```python
from build123d import *

# Parameters (mm, degrees)
F0_W           = 850
F0_H           = 1920
F0_W_2         = 810
F0_H_2         = 1880
F1_DEPTH       = 20
F2_W           = 850
F2_H           = 50
F3_DEPTH       = 10
F6_DEPTH       = 20
F8_DEPTH       = 10
F8_DEPTH_BACK  = 10
F10_DEPTH      = 20
F11_R          = 4.25
F12_DEPTH      = 960.001
F12_DEPTH_BACK = 960.001


with BuildPart() as f1:
    # F0 (on Top) → F1 (new body)
    with BuildSketch(Plane.XY):
        Rectangle(F0_W, F0_H)
        Rectangle(F0_W_2, F0_H_2, mode=Mode.SUBTRACT)
    extrude(amount=F1_DEPTH)

    # F2 (on face) → F3 (join)
    with BuildSketch(Plane.XY.offset(20)):
        with Locations((0, 785)):
            Rectangle(F2_W, F2_H)
        with Locations((0, 585)):
            Rectangle(F2_W, F2_H)
        with Locations((0, 385)):
            Rectangle(F2_W, F2_H)
        with Locations((0, 185)):
            Rectangle(F2_W, F2_H)
        with Locations((0, -15)):
            Rectangle(F2_W, F2_H)
        with Locations((0, -215)):
            Rectangle(F2_W, F2_H)
        with Locations((0, -415)):
            Rectangle(F2_W, F2_H)
        with Locations((0, -615)):
            Rectangle(F2_W, F2_H)
        with Locations((0, -815)):
            Rectangle(F2_W, F2_H)
    extrude(amount=F3_DEPTH)

    # F5 (on face) → F6 (join)
    with BuildSketch(Plane.XZ.offset(960)):
        Polygon((445, 180), (425, 180), (425, 0), (145, 0), (145, -20), (445, -20), align=None)
    extrude(amount=-F6_DEPTH)

    # F7 (on Front) → F8 (join, two sides)
    with BuildSketch(Plane.XZ) as f8_sk:
        Polygon((425, 0), (-425, 0), (-425, -20), (445, -20), (445, 180), (425, 180), align=None)
    extrude(amount=F8_DEPTH)
    extrude(f8_sk.sketch, amount=-F8_DEPTH_BACK)

    # F9 (on face) → F10 (join)
    with BuildSketch(Plane(origin=(0, 960, 0), x_dir=(-1, 0, 0), z_dir=(0, 1, 0))):
        Polygon((425, 0), (-425, 0), (-425, 180), (-445, 180), (-445, -20), (425, -20), align=None)
    extrude(amount=-F10_DEPTH)

    # F11 (on Front) → F12 (cut, two sides)
    with BuildSketch(Plane.XZ) as f12_sk:
        with Locations((435, 170)):
            Circle(F11_R)
    extrude(amount=-F12_DEPTH, mode=Mode.SUBTRACT)
    extrude(f12_sk.sketch, amount=F12_DEPTH_BACK, mode=Mode.SUBTRACT)


solid = f1.part
```
For this review, take the finished solid that the model builds, in its own axes (mm). A direction names the side the tool comes from. Round coordinates to 2 decimals unless told otherwise and drop trailing zeros. Write each loop counter-clockwise with the first axis right and the second up, starting at its lowest first coordinate (ties: lowest second). Pieces come first, ordered by that corner, then holes. Notation, with made-up numbers: (-1, 70.25) -> (4, 70.25) arc R14 ccw to (4, 89.25) -> close; hole circle Ø1 at (53, 11). An arc over 180 degrees is marked (long way). One line per question, with ' | ' between items. Start each with the question number.
(1) For line 1 along Z through (x, y) = (435, 4.75); line 2 along Y through (x, z) = (371.5, -8); line 3 along Y through (x, z) = (-254, -8.5), list the stretches that pass through material, from the lowest coordinate up. Write a range as from..to.
(2) Tool access review of faces 1 (the face through (-2, 941, 20)), 2 (the face through (-416, -694, 0)), 3 (the face through (-6, 185, 20)), 4 (the face through (-6, -15, 20)): name each direction out of +Z, -Z, +X, -X, +Y, -Y from which nothing blocks a thin tool from reaching the whole face with its end or side.
(3) Insertion check: P1, Ø16, axis at x = -418, y = -527, coming from the +Z side; P2, Ø3, axis at x = -35.5, z = 26.5, coming from the -Y side; P3, Ø6, axis at y = -237.5, z = 2, coming from the +X side. Each pin has a flat end and moves straight along its axis. Give the tip position at first contact, or say it passes through.
(4) Mouldability with a two-part tool opening along X and no side actions: class faces 5 (the face through (-2, -949, 20)), 6 (the face through (-6, -815, 20)), 7 (the face through (-425, -13, 11)) as released by +X, released by -X, zero draft, split by the parting line, or undercut.
(5) Add section A-A, the plane y = -294. Write out the cut boundary in (x, z), plus the area to 3 significant figures.
(6) Add section B-B, the plane z = 144.5. Write out the cut boundary in (x, y), plus the area to 3 significant figures.
(7) Add section C-C, the plane x = 324. Give the number of separate pieces and of enclosed holes in the cut face, plus the area to 3 significant figures.
Answer list:
1) line 1: -20..165.75, 174.25..180 | line 2: -960..-940, -10..10, 940..960 | line 3: -10..10, 940..960
2) face 1: +Z, -X, +Y | face 2: -Z, -X, -Y | face 3: -Z | face 4: none
3) P1: z = 20 | P2: y = -840 | P3: x = 425
4) face 5: zero draft | face 6: undercut | face 7: released by -X
5) outline: (-425, 0) -> (-405, 0) -> (-405, 20) -> (-425, 20) -> close; (405, 0) -> (425, 0) -> (425, 20) -> (405, 20) -> close | area: 800 mm²
6) outline: (425, -960) -> (445, -960) -> (445, -940) -> (425, -940) -> close; (425, -10) -> (445, -10) -> (445, 10) -> (425, 10) -> close; (425, 940) -> (445, 940) -> (445, 960) -> (425, 960) -> close | area: 1,200 mm²
7) separate pieces: 12 | enclosed holes: 0 | area: 6,500 mm²
